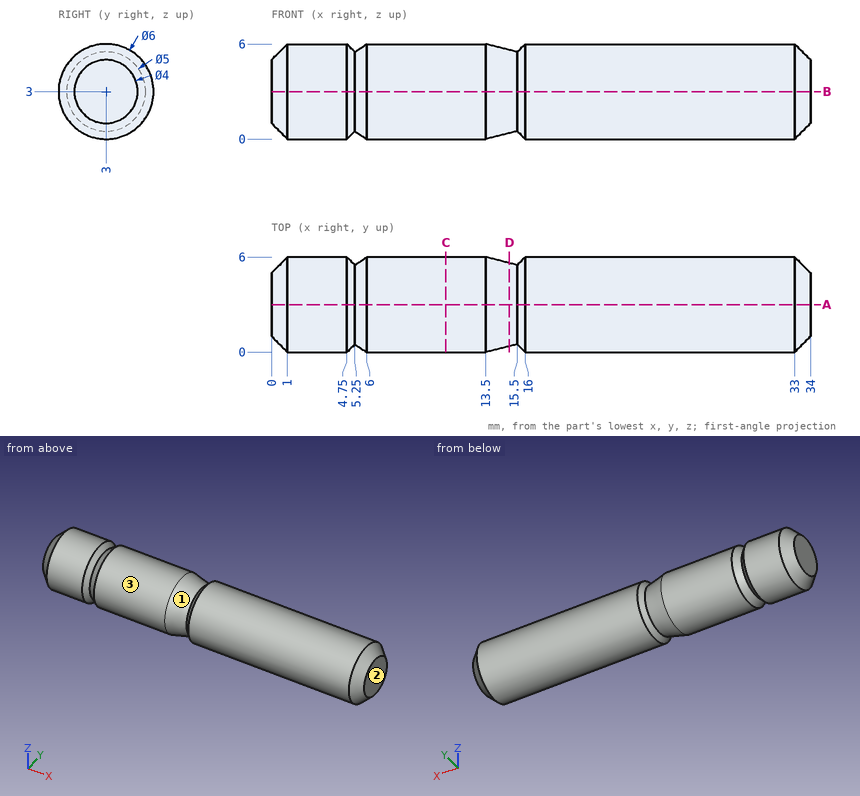
Here's the drawing with two shaded views (mm, measured from the low corner). I have some questions. Round coordinates to 2 decimals unless told otherwise and drop trailing zeros. Loops run counter-clockwise (first coordinate to the right, second up) from the corner with the lowest first, then second, coordinate; pieces in that order, holes last. Notation, with made-up numbers: (-33.75, 63) - (14.25, 63) arc R24 cw to (14.25, 77) - close; hole circle Ø5 at (-40, 76). An arc over 180 degrees is marked (long way). Use CSV: the item, a comma, the result in double quotes.
Item 1: If we mould it in two halves opening along X, with no side actions, what happens to the marked faces 1, 2 and 3? For each: pulls with the +X half, pulls with the -X half, needs draft (parallel to the pull), parting line crosses it, or undercut.
Here are the results:
face 1,"undercut"
face 2,"pulls with the +X half"
face 3,"needs draft"
Item 2: Will these pins go through, and if not, where does the flat tip stop? pin 1 (3 mm diameter, centred on y = 5, z = 0.5, fed in from +X); pin 2 (1 mm diameter, centred on x = 13, y = 5, fed in from +Z).
Here are the results:
pin 1,"stops at x = 34"
pin 2,"stops at z = 5.6"
Item 3: If we section it at C-C on x = 11: List the corners of the cut face in (y, z) for me.
Here are the results:
outline,"circle Ø6 at (3, 3)"
Item 4: If we section it at A-A on y = 3: List the corners of the cut face in (x, z) for me, then the cut area to 3 significant figures.
Here are the results:
outline,"(0, 1) - (1, 0) - (4.75, 0) - (5.25, 0.5) - (6, 0) - (13.5, 0) - (15.5, 0.5) - (16, 0) - (33, 0) - (34, 1) - (34, 5) - (33, 6) - (16, 6) - (15.5, 5.5) - (13.5, 6) - (6, 6) - (5.25, 5.5) - (4.75, 6) - (1, 6) - (0, 5) - close"
area,"200 mm²"
Item 5: I need wall thicknesses on L1, parallel to Y at x = 24.5, z = 2.8; L2, parallel to Y at x = 7, z = 3.9. Which ranges of each line are inside material? Lowest first, please. Write a range as [from, to].
Here are the results:
L1,"y = [0.01, 5.99]"
L2,"y = [0.14, 5.86]"
Item 6: If we section it at D-D on x = 15: List the corners of the cut face in (y, z) for me (3 decimals), then the cut area to 3 significant figures.
Here are the results:
outline,"circle Ø5.25 at (3, 3)"
area,"21.6 mm²"
